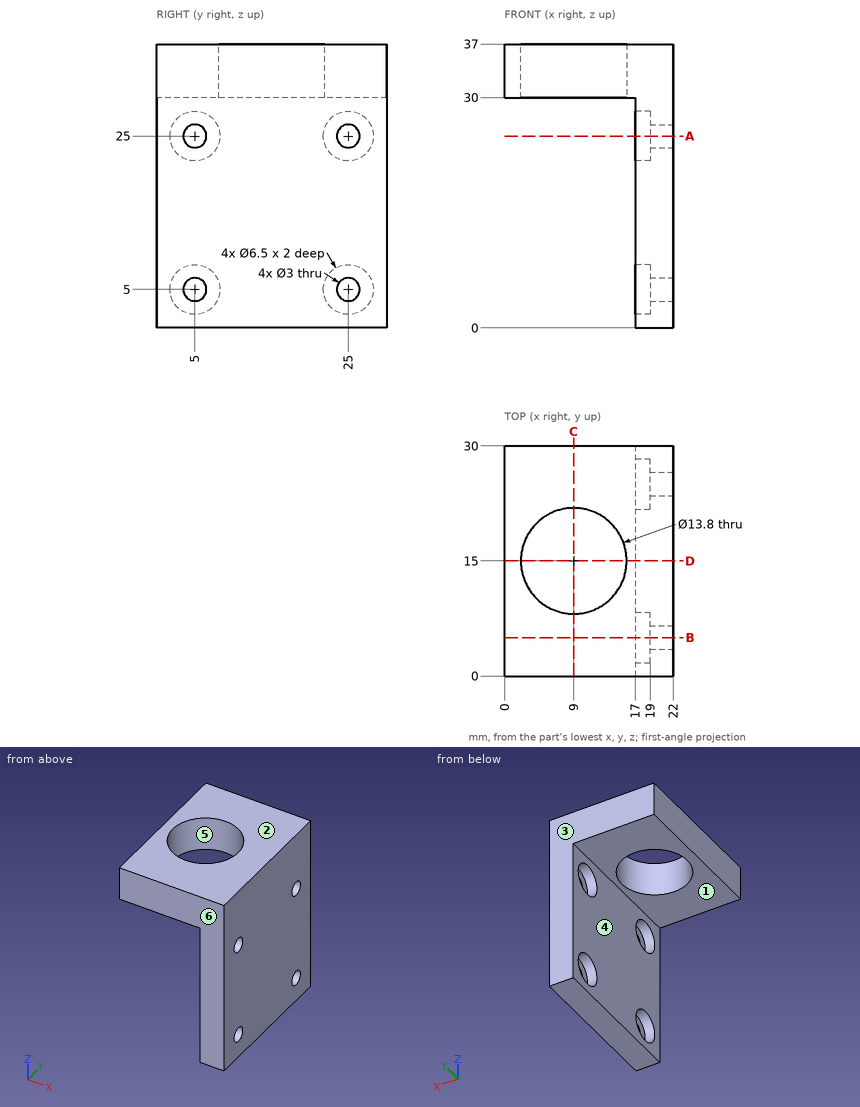
Study the drawing (mm; zero at the part's minimum x, y, z) and answer. A direction names the side the tool comes from. Give positions to 0.01 mm unless a question says otherwise; leave off trailing zeros. Loops run counter-clockwise (first coordinate to the right, second up) from the corner with the lowest first, then second, coordinate; pieces in that order, holes last. Notation, with made-up numbers: M -37.5,-32.75 L -28.5,-32.75 A26 ccw -28.5,3.25 Z; hole C 10,79.25 d10. An arc over 180 degrees is marked long. One line per item, written item: value.
1. For a pull along Y with two mould halves and no side action, classify the marked faces 3, 4, 5 and 6 as pulls with the +Y half, pulls with the -Y half, needs draft (parallel to the pull), parting line crosses it, or undercut.
Found:
face 3: pulls with the +Y half
face 4: needs draft
face 5: undercut
face 6: pulls with the -Y half
2. Each of these flat-tipped pins is pushed along its axis until it touches: P1, Ø5, axis at y = 5, z = 3.5, coming from the -X side; P2, Ø2, axis at y = 25.5, z = 6.5, coming from the -X side. Where does it stop, or does it pass through?
Found:
P1: x = 17
P2: x = 19
3. For the marked faces 1 and 2, determine the directions among +Z, -Z, +X, -X, +Y, -Y from which every point of the face is accessible in a straight line to the end or side of a thin tool.
Found:
face 1: -Z, -X, +Y, -Y
face 2: +Z, +X, -X, +Y, -Y
4. Section D-D on y = 15 is taken. Determine the outline of the cut face in (x, z).
Found:
outline: M 0,30 L 2.1,30 L 2.1,37 L 0,37 Z; M 15.9,30 L 17,30 L 17,0 L 22,0 L 22,37 L 15.9,37 Z
5. Find the intervals of material crossed by probe 1 along Z at (x, y) = (20.3, 25); probe 2 along Z at (x, y) = (17.45, 25); probe 3 along X at (y, z) = (27.75, 6.5), in increasing order.
Found:
probe 1: 0 to 3.5, 6.5 to 23.5, 26.5 to 37
probe 2: 0 to 1.75, 8.25 to 21.75, 28.25 to 37
probe 3: 19 to 22
6. Section C-C on x = 9 is taken. Determine the outline of the cut face in (y, z).
Found:
outline: M 0,30 L 8.1,30 L 8.1,37 L 0,37 Z; M 21.9,30 L 30,30 L 30,37 L 21.9,37 Z
7. Section A-A on z = 25 is taken. Determine the outline of the cut face in (x, y), plus the area to 3 significant figures.
Found:
outline: M 17,0 L 22,0 L 22,3.5 L 19,3.5 L 19,1.75 L 17,1.75 Z; M 17,8.25 L 19,8.25 L 19,6.5 L 22,6.5 L 22,23.5 L 19,23.5 L 19,21.75 L 17,21.75 Z; M 17,28.25 L 19,28.25 L 19,26.5 L 22,26.5 L 22,30 L 17,30 Z
area: 106 mm^2
8. Section B-B on y = 5 is taken. Determine the outline of the cut face in (x, z), plus the area to 3 significant figures.
Found:
outline: M 0,30 L 17,30 L 17,28.25 L 19,28.25 L 19,26.5 L 22,26.5 L 22,37 L 0,37 Z; M 17,0 L 22,0 L 22,3.5 L 19,3.5 L 19,1.75 L 17,1.75 Z; M 17,8.25 L 19,8.25 L 19,6.5 L 22,6.5 L 22,23.5 L 19,23.5 L 19,21.75 L 17,21.75 Z
area: 260 mm^2
